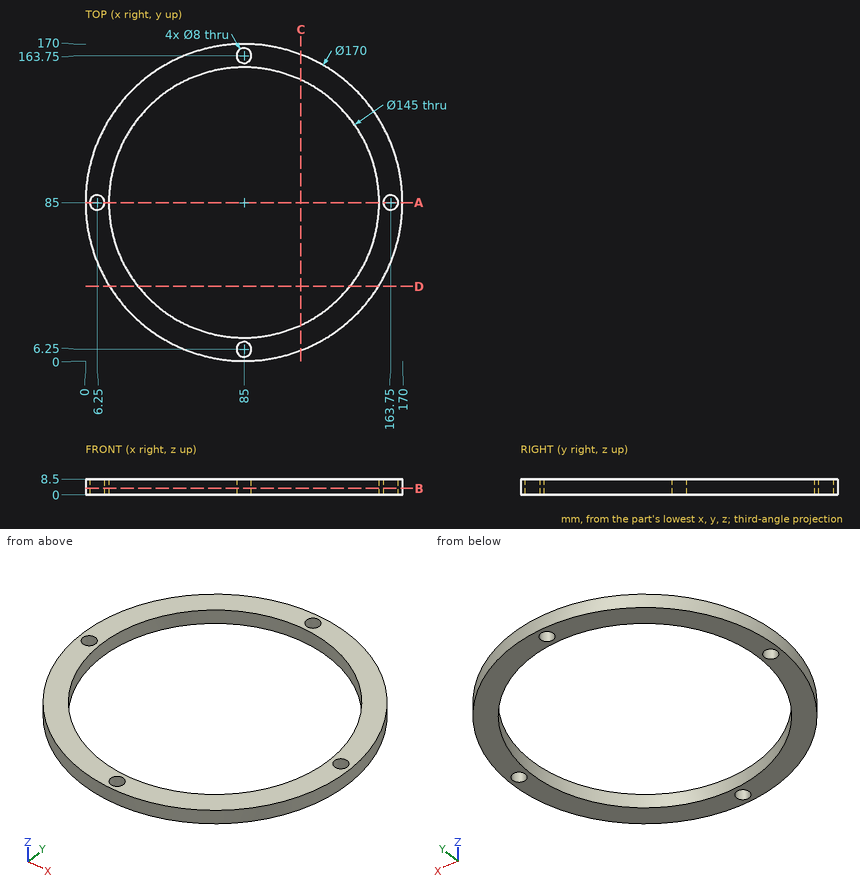
Answer from the drawing. Dimensions are ordinates in mm from the lowest x, y and z of the part. Round coordinates to 2 decimals unless told otherwise and drop trailing zeros. Order: outer loops, then holes, each group sorted by start corner. A loop starts at its lowest first (then second) coordinate and runs counter-clockwise, first axis right, second up. Notation, with made-up numbers: (-25, 76) - (18, 76) arc R32 ccw to (18, 104) - close; hole circle Ø3 at (9, -38). An arc over 180 degrees is marked (long way). Put each result on its own line as item: value. Start each with the question number.
(1) Straight lines are drawn through the part: probe 1 along Y at (x, z) = (85, 3); probe 2 along Y at (x, z) = (88.5, 4.25); probe 3 along X at (y, z) = (131.5, 3). For each, find the intervals that lie inside material, in ascending order. Write a range as from..to.
(2) Find section A-A (y = 85). Give the vertices of the cut face in (x, z), plus the area to 3 significant figures.
(3) Find section C-C (x = 115.5). Give the vertices of the cut face in (y, z), plus the area to 3 significant figures.
(4) Find section B-B (z = 3.5). Give the vertices of the cut face in (x, y).
(5) Find section D-D (y = 40). Give the vertices of the cut face in (x, z), plus the area to 3 significant figures.
(6) Given P1, Ø1.5, axis at y = 64.5, z = 3.5, coming from the +X side; P2, Ø9, axis at x = 163.75, y = 85, coming from the +Z side, each flat-ended and moving along its own axis, determine where each tip first touches the part or whether it passes through.
Reply:
1. probe 1: 0..2.25, 10.25..12.5, 157.5..159.75, 167.75..170
1. probe 2: 0.07..4.31, 8.19..12.58, 157.42..161.81, 165.69..169.93
1. probe 3: 13.85..29.38, 140.62..156.15
2. outline: (0, 0) - (2.25, 0) - (2.25, 8.5) - (0, 8.5) - close; (10.25, 0) - (12.5, 0) - (12.5, 8.5) - (10.25, 8.5) - close; (157.5, 0) - (159.75, 0) - (159.75, 8.5) - (157.5, 8.5) - close; (167.75, 0) - (170, 0) - (170, 8.5) - (167.75, 8.5) - close
2. area: 76.5 mm^2
3. outline: (5.66, 0) - (19.23, 0) - (19.23, 8.5) - (5.66, 8.5) - close; (150.77, 0) - (164.34, 0) - (164.34, 8.5) - (150.77, 8.5) - close
3. area: 231 mm^2
4. outline: circle Ø170 at (85, 85); hole circle Ø8 at (6.25, 85); hole circle Ø145 at (85, 85); hole circle Ø8 at (85, 6.25); hole circle Ø8 at (85, 163.75); hole circle Ø8 at (163.75, 85)
5. outline: (12.89, 0) - (28.16, 0) - (28.16, 8.5) - (12.89, 8.5) - close; (141.84, 0) - (157.11, 0) - (157.11, 8.5) - (141.84, 8.5) - close
5. area: 260 mm^2
6. P1: x = 167.67
6. P2: z = 8.5
